Read the model definition and answer for the solid it produces. Units are mm, in the model's axes. A direction names the side the tool comes from. Give positions to 0.01 mm unless a question says otherwise; leave off trailing zeros. Order: outer loops, then holes, each group sorted by start corner. A loop starts at its lowest first (then second) coordinate and runs counter-clockwise, first axis right, second up. Notation, with made-up numbers: (48.5, 29) -> (58.5, 29) arc R13 cw to (58.5, 54) -> close; hole circle Ø2 at (-8.5, 77). An arc over 180 degrees is marked (long way). One line per question, with ' | ' between items. Start each with the question number.
```python
from build123d import *

# Parameters (mm, degrees)
SKETCH1_R           = 4.7625
BOSS_EXTRUDE1_DEPTH = 97.3074
SKETCH3_R           = 9.078890277
SKETCH3_R_2         = 3.8481
CUT_EXTRUDE1_DEPTH  = 0.4445
SKETCH4_R           = 7.766517843
SKETCH4_R_2         = 3.8481
CUT_EXTRUDE2_DEPTH  = 0.4445
SKETCH5_R           = 6.35
CUT_EXTRUDE3_DEPTH  = 5.5118
SKETCH6_R           = 6.35
CUT_EXTRUDE4_DEPTH  = 3.5941


with BuildPart() as part:
    # Sketch1 → Boss-Extrude1 (new body)
    with BuildSketch(Plane.XY):
        Circle(SKETCH1_R)
    extrude(amount=BOSS_EXTRUDE1_DEPTH)

    # Sketch3 → Cut-Extrude1 (cut, symmetric)
    with BuildSketch(Plane(origin=(0, 0, 7.2136), x_dir=(-1, 0, 0), z_dir=(0, 0, -1))):
        Circle(SKETCH3_R)
        Circle(SKETCH3_R_2, mode=Mode.SUBTRACT)
    extrude(amount=CUT_EXTRUDE1_DEPTH, both=True, mode=Mode.SUBTRACT)

    # Sketch4 → Cut-Extrude2 (cut, symmetric)
    with BuildSketch(Plane.XY.offset(88.6206)):
        Circle(SKETCH4_R)
        Circle(SKETCH4_R_2, mode=Mode.SUBTRACT)
    extrude(amount=CUT_EXTRUDE2_DEPTH, both=True, mode=Mode.SUBTRACT)

    # Sketch5 → Cut-Extrude3 (cut)
    with BuildSketch(Plane.XY.offset(97.3074)):
        Circle(SKETCH5_R)
    extrude(amount=-CUT_EXTRUDE3_DEPTH, mode=Mode.SUBTRACT)

    # Sketch6 → Cut-Extrude4 (cut)
    with BuildSketch(Plane(origin=(0, 0, 0), x_dir=(-1, 0, 0), z_dir=(0, 0, -1))):
        Circle(SKETCH6_R)
    extrude(amount=-CUT_EXTRUDE4_DEPTH, mode=Mode.SUBTRACT)


solid = part.part
```
Q1. Find the intervals of material crossed by line 1 (Z direction, x = 2.75, y = -2.75); line 2 (X direction, y = -0.25, z = 75.5); line 3 (X direction, y = -2, z = 46), in increasing order.
Q2. Determine the mould class of faces 3 (the flat face through (4, 0, 88.176)), 4 (the flat face through (0, 0, 91.796)), 5 (the cylindrical face through (-3.78, -2.9, 47.35)) for opening direction Z: pulls with the +Z half, pulls with the -Z half, needs draft (parallel to the pull), parting line crosses it, or undercut.
Q3. A cutting plane is placed at B-B, the plane x = -3. Determine the outline of the cut face in (y, z), then the cut area to 3 significant figures.
Q4. A cutting plane is placed at A-A, the plane y = -2.5. Determine the outline of the cut face in (x, z).
Q5. Given P1, Ø5, axis at y = 3.5, z = 48.5, coming from the -X side; P2, Ø1, axis at x = 2.5, z = 31.5, coming from the +Y side; P3, Ø1.5, axis at y = 3.5, z = 65, coming from the -X side, each flat-ended and moving along its own axis, determine where each tip first touches the part or whether it passes through.
Q6. A cutting plane is placed at C-C, the plane z = 85.5. Determine the outline of the cut face in (x, y) (1 decimal).
Q7. Which of the six approach directions +Z, -Z, +X, -X, +Y, -Y give full straight-line access (tool end or side, diameter ignored) to faces 1 (the cylindrical face through (-0.834, -3.757, 88.614)), 2 (the cylindrical face through (-3.78, -2.9, 5.16))?
Geometry results:
1) line 1: 3.59 to 6.77, 7.66 to 88.18, 89.07 to 91.8 | line 2: -4.76 to 4.76 | line 3: -4.32 to 4.32
2) face 3: undercut | face 4: pulls with the +Z half | face 5: needs draft
3) outline: (-3.7, 3.59) -> (3.7, 3.59) -> (3.7, 6.77) -> (2.41, 6.77) -> (2.41, 7.66) -> (3.7, 7.66) -> (3.7, 88.18) -> (2.41, 88.18) -> (2.41, 89.07) -> (3.7, 89.07) -> (3.7, 91.8) -> (-3.7, 91.8) -> (-3.7, 89.07) -> (-2.41, 89.07) -> (-2.41, 88.18) -> (-3.7, 88.18) -> (-3.7, 7.66) -> (-2.41, 7.66) -> (-2.41, 6.77) -> (-3.7, 6.77) -> close | area: 648 mm²
4) outline: (-4.05, 3.59) -> (4.05, 3.59) -> (4.05, 6.77) -> (2.93, 6.77) -> (2.93, 7.66) -> (4.05, 7.66) -> (4.05, 88.18) -> (2.93, 88.18) -> (2.93, 89.07) -> (4.05, 89.07) -> (4.05, 91.8) -> (-4.05, 91.8) -> (-4.05, 89.07) -> (-2.93, 89.07) -> (-2.93, 88.18) -> (-4.05, 88.18) -> (-4.05, 7.66) -> (-2.93, 7.66) -> (-2.93, 6.77) -> (-4.05, 6.77) -> close
5) P1: x = -4.66 | P2: y = 4.32 | P3: x = -3.89
6) outline: circle Ø9.5 at (0, 0)
7) face 1: none | face 2: +Z, -Z
